Could you check a few things on this model? Use its own coordinates, in mm. Face numbers are marked on the shaded views. A direction names the side the tool comes from. Round coordinates to 2 decimals unless told otherwise and drop trailing zeros. Loops run counter-clockwise (first coordinate to the right, second up) from the corner with the lowest first, then second, coordinate; pieces in that order, holes last. Notation, with made-up numbers: (79, 67) - (133, 67) arc R27 cw to (133, 87) - close; hole circle Ø6 at (10, 63.25). An arc over 180 degrees is marked (long way). Use one line per item in the form item = value.
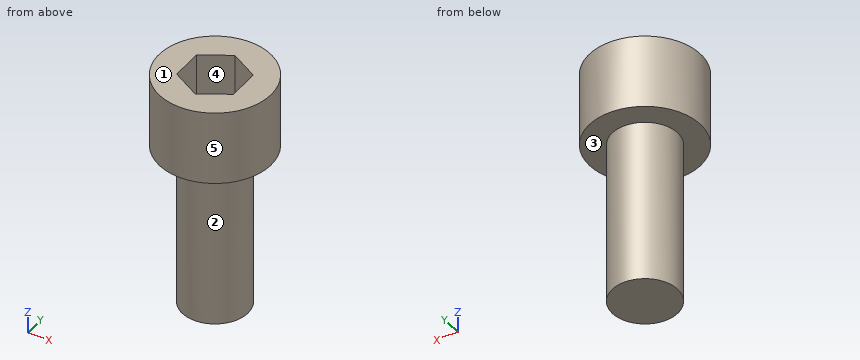
```python
from build123d import *

# Parameters (mm, degrees)
SKETCH_1_R      = 2
EXTRUDE_1_DEPTH = 10
SKETCH_2_R      = 3.4
EXTRUDE_2_DEPTH = 4.5


with BuildPart() as part:
    # 草图1 → 拉伸1 (new body)
    with BuildSketch(Plane.XY):
        Circle(SKETCH_1_R)
    extrude(amount=EXTRUDE_1_DEPTH)

    # 草图2 → 拉伸2 (add)
    with BuildSketch(Plane.XY.offset(10)):
        Circle(SKETCH_2_R)
        Polygon((-0.031811461, 1.981453179), (-1.73189452, 0.963177056), (-1.700083059, -1.018276123), (0.031811461, -1.981453179), (1.73189452, -0.963177056), (1.700083059, 1.018276123), align=None, mode=Mode.SUBTRACT)
    extrude(amount=EXTRUDE_2_DEPTH)


solid = part.part
```
1. We'd pull the mould along X, two halves only. Please class the marked faces 3, 4 and 5: +X half, -X half, draft (parallel to the pull), parting line (faces both ways), or undercut.
Solution:
face_3 = draft
face_4 = undercut
face_5 = parting line
2. If we section it at C-C, the plane y = -1.75: Write out the boundary of the cut face in (x, z), plus the area to 3 significant figures.
Solution:
outline = (-2.92, 10) - (-0.97, 10) - (-0.97, 0) - (0.97, 0) - (0.97, 10) - (2.92, 10) - (2.92, 14.5) - (0.42, 14.5) - (0.42, 10) - (-0.38, 10) - (-0.38, 14.5) - (-2.92, 14.5) - close
area = 42.0 mm^2
3. On a 3-axis mill with a long thin cutter (end or side, diameter ignored), from which of +Z, -Z, +X, -X, +Y, -Y can I reach the whole of each face in a straight line? I mean the marked faces 1 and 2. Say none if no direction works.
Solution:
face_1 = +Z, +X, -X, +Y, -Y
face_2 = -Z
4. For P1, Ø4, axis at x = -0.5, y = -1, coming from the +Z side; P2, Ø1.5, axis at x = -0.5, z = 1.5, coming from the -Y side; P3, Ø1.5, axis at y = -1, z = 7, coming from the +X side, each with a flat end and sliding along its axis, tell me the tip position at first contact or that it passes through.
Solution:
P1 = 14.5
P2 = -2
P3 = 1.98
5. If we section it at D-D, the plane z = 2: Write out the boundary of the cut face in (x, y), plus the area to 3 significant figures.
Solution:
outline = circle Ø4 at (0, 0)
area = 12.6 mm^2
6. If we section it at A-A, the plane z = 12.5: Write out the boundary of the cut face in (x, y), plus the area to 3 significant figures.
Solution:
outline = circle Ø6.8 at (0, 0); hole (-1.73, 0.96) - (-1.7, -1.02) - (0.03, -1.98) - (1.73, -0.96) - (1.7, 1.02) - (-0.03, 1.98) - close
area = 26.1 mm^2
7. If we section it at B-B, the plane x = 1.25: Write out the boundary of the cut face in (y, z), plus the area to 3 significant figures.
Solution:
outline = (-3.16, 10) - (-1.56, 10) - (-1.56, 0) - (1.56, 0) - (1.56, 10) - (3.16, 10) - (3.16, 14.5) - (1.27, 14.5) - (1.27, 10) - (-1.25, 10) - (-1.25, 14.5) - (-3.16, 14.5) - close
area = 48.3 mm^2
8. Please list where these lines run through material, in increasing order: line 1 along Z through (x, y) = (-1.75, 1.5); line 2 along Z through (x, y) = (-1, 0); line 3 along Y through (x, z) = (-2.75, 12.5).
Solution:
line_1 = 10 to 14.5
line_2 = 0 to 10
line_3 = -2 to 2
